```python
from build123d import *
from OCP.BRepFilletAPI import BRepFilletAPI_MakeChamfer

# Parameters (mm, degrees)
SKETCH1_W           = 43.942
SKETCH1_H           = 18.542
BOSS_EXTRUDE1_DEPTH = 7.62
CHAMFER1_SIZE       = 10.910412501
CHAMFER1_SIZE_2     = 0.381
SHELL1_T            = -2.54
SKETCH2_W           = 50.8
SKETCH2_H           = 25.4
BOSS_EXTRUDE2_DEPTH = 5.08
CHAMFER2_SIZE       = 2.54
CHAMFER2_SIZE2      = 11.949760478
FILLET1_R           = 2.54


with BuildPart() as part:
    # Sketch1 → Boss-Extrude1 (new body)
    with BuildSketch(Plane(origin=(0, 0, 0), x_dir=(1, 0, 0), z_dir=(0, 1, 0))):
        Rectangle(SKETCH1_W, SKETCH1_H)
    extrude(amount=BOSS_EXTRUDE1_DEPTH)

    # Chamfer1
    # the kernel refuses this chamfer: 10.910412501, 0.381 mm, written as the material it takes off along each edge
    with BuildSketch(Plane(origin=(-21.971, 0, 37.637433425), x_dir=(-0.0013423185755923317, 0.999999099090015, 0), z_dir=(0, 0, -1)), Plane(origin=(21.971, 0, -37.637433425), x_dir=(0.0013423185755923317, 0.999999099090015, 0), z_dir=(0, 0, 1))) as chamfer1_piece_1:
        Polygon((CHAMFER1_SIZE * 0.999999099071, CHAMFER1_SIZE * 0.00134231857557), (-CHAMFER1_SIZE_2 * 0.00134231857559, CHAMFER1_SIZE_2 * 0.99999909909), (0, 0), align=None)
    extrude(amount=75.27486685, mode=Mode.SUBTRACT)
    with BuildSketch(Plane(origin=(-50.337433425, 0, -9.271), x_dir=(0, 0.999999099090015, -0.0013423185755923317), z_dir=(1, 0, 0)), Plane(origin=(50.337433425, 0, 9.271), x_dir=(0, 0.999999099090015, 0.0013423185755923317), z_dir=(-1, 0, 0))) as chamfer1_piece_2:
        Polygon((CHAMFER1_SIZE * 0.999999099071, CHAMFER1_SIZE * 0.00134231857557), (-CHAMFER1_SIZE_2 * 0.00134231857559, CHAMFER1_SIZE_2 * 0.99999909909), (0, 0), align=None)
    extrude(amount=100.67486685, mode=Mode.SUBTRACT)

    # Shell1
    shell1_openings = [part.faces().sort_by_distance(p)[0] for p in [
        (0, 0, 0),
    ]]
    offset(amount=SHELL1_T, openings=shell1_openings, kind=Kind.INTERSECTION)

    # Sketch2 → Boss-Extrude2 (add)
    with BuildSketch(Plane(origin=(0, 7.62, 0), x_dir=(1, 0, 0), z_dir=(0, 1, 0))):
        Rectangle(SKETCH2_W, SKETCH2_H)
    extrude(amount=BOSS_EXTRUDE2_DEPTH)

    # Chamfer2: one chamfer whose edges measure the first distance from different faces: ONE call of the kernel's chamfer builder (chamfer() names one face for all edges)
    chamfer2_edges_1 = [part.edges().sort_by_distance(p)[0] for p in [
        (-25.4, 12.7, 0),
    ]]
    chamfer2_side_1 = [part.faces().sort_by_distance(p)[0] for p in [
        (-25.4, 10.16, 0),
    ]]
    chamfer2_edges_2 = [part.edges().sort_by_distance(p)[0] for p in [
        (0, 12.7, 12.7),
    ]]
    chamfer2_side_2 = [part.faces().sort_by_distance(p)[0] for p in [
        (0, 10.16, 12.7),
    ]]
    chamfer2_edges_3 = [part.edges().sort_by_distance(p)[0] for p in [
        (25.4, 12.7, 0),
    ]]
    chamfer2_side_3 = [part.faces().sort_by_distance(p)[0] for p in [
        (25.4, 10.16, 0),
    ]]
    chamfer2_edges_4 = [part.edges().sort_by_distance(p)[0] for p in [
        (0, 12.7, -12.7),
    ]]
    chamfer2_side_4 = [part.faces().sort_by_distance(p)[0] for p in [
        (0, 10.16, -12.7),
    ]]
    chamfer2 = BRepFilletAPI_MakeChamfer(part.part.solid().wrapped)
    for e in chamfer2_edges_1:
        chamfer2.Add(CHAMFER2_SIZE, CHAMFER2_SIZE2, e.wrapped, chamfer2_side_1[0].wrapped)  # the first distance lies on this face
    for e in chamfer2_edges_2:
        chamfer2.Add(CHAMFER2_SIZE, CHAMFER2_SIZE2, e.wrapped, chamfer2_side_2[0].wrapped)  # the first distance lies on this face
    for e in chamfer2_edges_3:
        chamfer2.Add(CHAMFER2_SIZE, CHAMFER2_SIZE2, e.wrapped, chamfer2_side_3[0].wrapped)  # the first distance lies on this face
    for e in chamfer2_edges_4:
        chamfer2.Add(CHAMFER2_SIZE, CHAMFER2_SIZE2, e.wrapped, chamfer2_side_4[0].wrapped)  # the first distance lies on this face
    add(Compound.cast(chamfer2.Shape()), mode=Mode.REPLACE)

    # Fillet1
    fillet1_edges = [part.edges().sort_by_distance(p)[0] for p in [
        (0, 10.16, 12.7),
        (-25.4, 10.16, 0),
        (0, 10.16, -12.7),
        (25.4, 10.16, 0),
    ]]
    fillet(fillet1_edges, radius=FILLET1_R)


solid = part.part
```
Can you work these out from the model? Positions are in its coordinate system, mm. A direction names the side the tool comes from. Coordinates: 2 decimals unless noted, no trailing zeros. Loops run counter-clockwise (first coordinate to the right, second up) from the corner with the lowest first, then second, coordinate; pieces in that order, holes last. Notation, with made-up numbers: (-7, -25) -> (4, -25) arc R13 cw to (4, -18) -> close; hole circle Ø7 at (69, 88). An arc over 180 degrees is marked (long way). Answer as a JSON object with one key per item and string values.
1) For P1, Ø1, axis at x = -4, y = 4, coming from the -Z side; P2, Ø4, axis at x = -6.5, z = -1, coming from the -Y side; P3, Ø2, axis at x = 14, y = 6, coming from the +Z side, each with a flat end and sliding along its axis, tell me the tip position at first contact or that it passes through.
Results:
{"P1": "stops at z = -9.05", "P2": "stops at y = 5.08", "P3": "stops at z = 9.13"}
2) For faces 4 (the face through (0.36, 9.68, -12.15)), 5 (the face through (0, 7.62, 11)), which set-ups out of +Z, -Z, +X, -X, +Y, -Y let a thin tool reach every point of the face, with its end or its side?
Results:
{"face 4": "-Z, +X, -X, +Y", "face 5": "-Y"}
3) Imagine slicing it at A-A (x = -5). Please give me the cut outline in (y, z).
Results:
{"outline": "(0, -8.89) -> (7.62, -9.16) -> (7.62, -12.7) -> (8.1, -12.7) arc R2.54 ccw to (10.59, -10.69) -> (12.7, -0.75) -> (12.7, 0.75) -> (10.59, 10.69) arc R2.54 ccw to (8.1, 12.7) -> (7.62, 12.7) -> (7.62, 9.16) -> (0, 8.89) -> (0, 6.35) -> (5.08, 6.53) -> (5.08, -6.53) -> (0, -6.35) -> close"}
4) Imagine slicing it at C-C (z = 8.25). Please give me the cut outline in (x, y), then the cut area to 3 significant figures.
Results:
{"outline": "(-25.4, 7.62) -> (-21.86, 7.62) -> (-21.59, 0) -> (21.59, 0) -> (21.86, 7.62) -> (25.4, 7.62) -> (25.4, 8.1) arc R2.54 ccw to (23.39, 10.59) -> (20.95, 11.11) -> (-20.95, 11.11) -> (-23.39, 10.59) arc R2.54 ccw to (-25.4, 8.1) -> close", "area": "502 mm^2"}
5) Imagine slicing it at B-B (y = 3.5). Please give me the cut outline in (x, z).
Results:
{"outline": "(-21.71, -9.01) -> (21.71, -9.01) -> (21.71, 9.01) -> (-21.71, 9.01) -> close; hole (-19.17, -6.47) -> (19.17, -6.47) -> (19.17, 6.47) -> (-19.17, 6.47) -> close"}
6) Imagine slicing it at D-D (x = -16.5). Please give me the cut outline in (y, z), then the cut area to 3 significant figures.
Results:
{"outline": "(0, -8.89) -> (7.62, -9.16) -> (7.62, -12.7) -> (8.1, -12.7) arc R2.54 ccw to (10.59, -10.69) -> (12.05, -3.8) -> (12.05, 3.8) -> (10.59, 10.69) arc R2.54 ccw to (8.1, 12.7) -> (7.62, 12.7) -> (7.62, 9.16) -> (0, 8.89) -> (0, 6.35) -> (5.08, 6.53) -> (5.08, -6.53) -> (0, -6.35) -> close", "area": "166 mm^2"}
7) If I drill on line 1 (Z direction, x = -9, y = 1); line 2 (X direction, y = 1.5, z = -0.75); line 3 (Z direction, x = -12, y = 4.5), over which ranges is the centre line in solid material (lowest first)?
Results:
{"line 1": "z = -8.92 to -6.38, 6.38 to 8.92", "line 2": "x = -21.64 to -19.1, 19.1 to 21.64", "line 3": "z = -9.05 to -6.51, 6.51 to 9.05"}
8) Thinking about a two-plate mould opening in Z: for faces 1 (the face through (0, 5.08, 0)), 2 (the face through (19.454, 11.424, 0.15)), 3 (the face through (0.36, 9.68, 12.15)), which applies, pulls with the +Z half, pulls with the -Z half, needs draft (parallel to the pull), parting line crosses it, or undercut?
Results:
{"face 1": "undercut", "face 2": "needs draft", "face 3": "pulls with the +Z half"}
